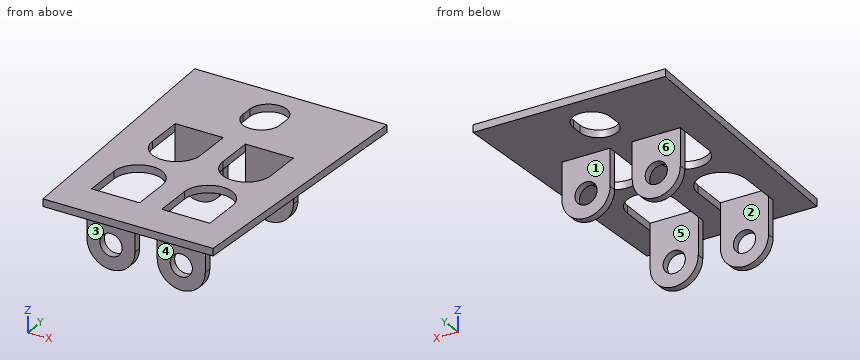
from build123d import *

# Parameters (mm, degrees)
EXTRUDE_1_DEPTH = 2
SKETCH_2_R      = 3
EXTRUDE_2_DEPTH = 2


with BuildPart() as part:
    # 草图1 → 凸台-拉伸1 (new body)
    with BuildSketch(Plane.XY):
        Polygon((-45.669718709, -55.644277912), (-48.669718709, 16.355722088), (3.330281291, 16.355722088), (0.330281291, -55.644277912), align=None)
        with BuildLine():
            ThreePointArc((-25.669718709, -35.644277912), (-32.169718709, -29.144277912), (-38.669718709, -35.644277912))
            Line((-38.669718709, -35.644277912), (-38.669718709, -45.644277912))
            Line((-38.669718709, -45.644277912), (-25.669718709, -45.644277912))
            Line((-25.669718709, -45.644277912), (-25.669718709, -35.644277912))
        make_face(mode=Mode.SUBTRACT)
        with BuildLine():
            ThreePointArc((-19.669718709, -18.644277912), (-13.169718709, -25.144277912), (-6.669718709, -18.644277912))
            Line((-6.669718709, -18.644277912), (-6.669718709, -8.644277912))
            Line((-6.669718709, -8.644277912), (-19.669718709, -8.644277912))
            Line((-19.669718709, -8.644277912), (-19.669718709, -18.644277912))
        make_face(mode=Mode.SUBTRACT)
        with BuildLine():
            ThreePointArc((-17.669718709, 6.355722088), (-22.669718709, 11.355722088), (-27.669718709, 6.355722088))
            Line((-27.669718709, 6.355722088), (-27.669718709, 3.355722088))
            ThreePointArc((-27.669718709, 3.355722088), (-22.669718709, -1.644277912), (-17.669718709, 3.355722088))
            Line((-17.669718709, 3.355722088), (-17.669718709, 6.355722088))
        make_face(mode=Mode.SUBTRACT)
        with BuildLine():
            Line((-25.669718709, -8.644277912), (-25.669718709, -18.644277912))
            ThreePointArc((-25.669718709, -18.644277912), (-32.169718709, -25.144277912), (-38.669718709, -18.644277912))
            Line((-38.669718709, -18.644277912), (-38.669718709, -8.644277912))
            Line((-38.669718709, -8.644277912), (-25.669718709, -8.644277912))
        make_face(mode=Mode.SUBTRACT)
        with BuildLine():
            Line((-19.669718709, -45.644277912), (-19.669718709, -35.644277912))
            ThreePointArc((-19.669718709, -35.644277912), (-13.169718709, -29.144277912), (-6.669718709, -35.644277912))
            Line((-6.669718709, -35.644277912), (-6.669718709, -45.644277912))
            Line((-6.669718709, -45.644277912), (-19.669718709, -45.644277912))
        make_face(mode=Mode.SUBTRACT)
    extrude(amount=EXTRUDE_1_DEPTH)

    # 草图2 → 凸台-拉伸2 (add)
    # profile 1 of 2: a face of its own
    with BuildSketch(Plane(origin=(0, -8.644277912, 0), x_dir=(-1, 0, 0), z_dir=(0, -1, 0))):
        with BuildLine():
            ThreePointArc((25.669718709, 10), (32.169718709, 16.5), (38.669718709, 10))
            Line((38.669718709, 10), (38.669718709, 0))
            Line((38.669718709, 0), (25.669718709, 0))
            Line((25.669718709, 0), (25.669718709, 10))
        make_face()
        with Locations(Location((32.169718709, 10, 0), (0, 0, 180))):
            Circle(SKETCH_2_R, mode=Mode.SUBTRACT)
    # profile 2 of 2: a face of its own
    with BuildSketch(Plane(origin=(0, -8.644277912, 0), x_dir=(-1, 0, 0), z_dir=(0, -1, 0))):
        with BuildLine():
            ThreePointArc((6.669718709, 10), (13.169718709, 16.5), (19.669718709, 10))
            Line((19.669718709, 10), (19.669718709, 0))
            Line((19.669718709, 0), (6.669718709, 0))
            Line((6.669718709, 0), (6.669718709, 10))
        make_face()
        with Locations(Location((13.169718709, 10, 0), (0, 0, 180))):
            Circle(SKETCH_2_R, mode=Mode.SUBTRACT)
    extrude_2 = extrude(amount=-EXTRUDE_2_DEPTH)

    # 镜向2: 凸台-拉伸2 across plane
    add(extrude_2.mirror(Plane(origin=(0, -27.144277912, 0), x_dir=(0, 0, 1), z_dir=(0, -1, 0))))


solid = part.part
Build history of the part. All positions in model axes, mm. Face numbers are marked on the shaded views. A direction names the side the tool comes from. Coordinates: 2 decimals unless noted, no trailing zeros. Write each loop counter-clockwise with the first axis right and the second up, starting at its lowest first coordinate (ties: lowest second). Pieces come first, ordered by that corner, then holes.
(1) Cut at C-C on y = -12. List the corners of the cut face in (x, z).
(2) Cut at D-D on z = -12. State how many separate pieces and enclosed holes the cut face has, and give its area (3 significant figures).
(3) 3-axis set-ups, long thin cutter, end or side, ignore diameter. For the marked faces 4, 5 and 6: which of +Z, -Z, +X, -X, +Y, -Y reach the whole face in a straight line?
(4) Pin check, flat tips, straight feed: pin 1 Ø2 at (y, z) = (-8, -3.5) entering from +X; pin 2 Ø10.5 at (x, z) = (-33, -8) entering from +Y; pin 3 Ø6 at (x, y) = (-10, -30) entering from -Z; pin 4 Ø1.5 at (x, z) = (-23.5, -6.5) entering from -Y. Stop position of each tip, or through.
(5) Drill centre lines: line 1 (Y direction, x = -35, z = -15.5); line 2 (Y direction, x = -31.5, z = 0.5); line 3 (Z direction, x = -37, y = 10). Where is each one in solid material? Low to high.
(6) Cut at B-B on x = -8.5. List the corners of the cut face in (y, z), and give its area (3 significant figures).
(7) Mould opens along Y. For the marked faces 1, 2 and 3 say: pulls with the +Y half, pulls with the -Y half, needs draft (parallel to the pull), parting line crosses it, or undercut.
(8) Cut at A-A on z = -6. List the corners of the cut face in (x, y), and give its area (3 significant figures).
Working result:
1. outline: (-47.49, 0) - (-38.67, 0) - (-38.67, 2) - (-47.49, 2) - close; (-25.67, 0) - (-19.67, 0) - (-19.67, 2) - (-25.67, 2) - close; (-6.67, 0) - (2.15, 0) - (2.15, 2) - (-6.67, 2) - close
2. separate pieces: 8
2. enclosed holes: 0
2. area: 63.2 mm2
3. face 4: -Z, +X, -X, -Y
3. face 5: +Z, -Z
3. face 6: -Z, +X, -X, +Y
4. pin 1: stops at x = -6.67
4. pin 2: stops at y = -6.64
4. pin 3: stops at z = 0
4. pin 4: passes through
5. line 1: y = -47.64 to -45.64, -8.64 to -6.64
5. line 2: y = -55.64 to -45.64, -29.18 to -25.11, -8.64 to 16.36
5. line 3: z = 0 to 2
6. outline: (-55.64, 0) - (-47.64, 0) - (-47.64, -14.52) - (-45.64, -14.52) - (-45.64, 2) - (-55.64, 2) - close; (-31.12, 0) - (-23.17, 0) - (-23.17, 2) - (-31.12, 2) - close; (-8.64, -14.52) - (-6.64, -14.52) - (-6.64, 0) - (16.36, 0) - (16.36, 2) - (-8.64, 2) - close
6. area: 144 mm2
7. face 1: pulls with the +Y half
7. face 2: undercut
7. face 3: pulls with the -Y half
8. outline: (-38.67, -47.64) - (-25.67, -47.64) - (-25.67, -45.64) - (-38.67, -45.64) - close; (-38.67, -8.64) - (-25.67, -8.64) - (-25.67, -6.64) - (-38.67, -6.64) - close; (-19.67, -47.64) - (-6.67, -47.64) - (-6.67, -45.64) - (-19.67, -45.64) - close; (-19.67, -8.64) - (-6.67, -8.64) - (-6.67, -6.64) - (-19.67, -6.64) - close
8. area: 104 mm2
